For this review, take the finished solid that the model builds, in its own axes (mm). Face numbers are marked on the shaded views. A direction names the side the tool comes from. Round coordinates to 2 decimals unless told otherwise and drop trailing zeros. Order: outer loops, then holes, each group sorted by start corner. A loop starts at its lowest first (then second) coordinate and runs counter-clockwise, first axis right, second up.
from build123d import *

# Parameters (mm, degrees)
BOSS_EXTRUDE1_DEPTH = 13.49375
BOSS_EXTRUDE2_DEPTH = 17.4625


with BuildPart() as part:
    # Sketch1 → Boss-Extrude1 (new body, symmetric)
    with BuildSketch(Plane.XY):
        Polygon((50.8, 0), (-50.8, 0), (-50.8, 34.925), (12.7, 51.939773719), (50.8, 29.942728463), align=None)
    extrude(amount=BOSS_EXTRUDE1_DEPTH, both=True)

    # Sketch2 → Boss-Extrude2 (add)
    with BuildSketch(Plane.XY.offset(13.49375)):
        Polygon((-50.8, 0), (-50.8, 34.925), (0, 21.313181024), (0, 0), align=None)
    extrude(amount=BOSS_EXTRUDE2_DEPTH)


solid = part.part
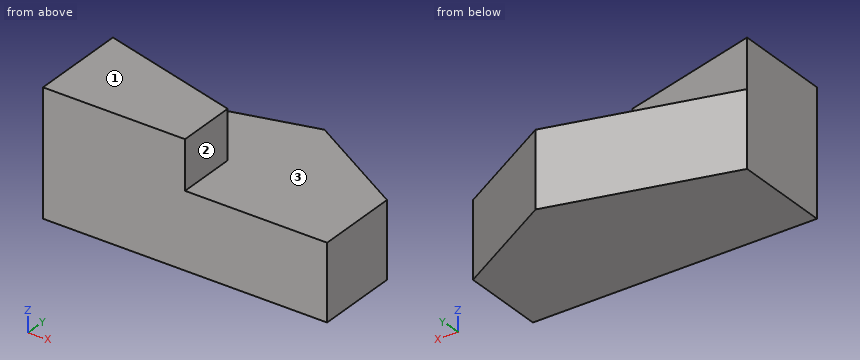
(1) Tool access review of the marked faces 1, 2 and 3: name each direction out of +Z, -Z, +X, -X, +Y, -Y from which nothing blocks a thin tool from reaching the whole face with its end or side.
(2) Add section D-D on x = 15.5. Give the boundary of the cut face in (y, z).
(3) Add section C-C on x = -38. Give the boundary of the cut face in (y, z), plus the area to 3 significant figures.
(4) Clearance check with flat-ended pins moving along their axes: P1, Ø12, axis at y = 39, z = 25.5, coming from the -X side; P2, Ø8.5, axis at y = 7, z = 25, coming from the +X side; P3, Ø10, axis at x = 2.5, y = 30, coming from the +Z side. State where each tip first meets the part, or that it passes through.
(5) Add section B-B on y = 10.5. Give the boundary of the cut face in (x, z), plus the area to 3 significant figures.
(6) Wall thickness on L1, parallel to X at y = 12.5, z = 26.5; L2, parallel to Z at x = 32, y = 11.5; L3, parallel to Y at x = 17.5, z = 13: over which ranges is each line inside the solid? List them lowest first.
(7) Add section A-A on z = -5.5. Give the boundary of the cut face in (x, y) (3 decimals).
Here are the results:
1. face 1: +Z, +X, -X, +Y, -Y
1. face 2: +Z, +X, +Y, -Y
1. face 3: +Z, +X, +Y
2. outline: (0, -13.49) - (50.32, -13.49) - (50.32, 13.49) - (0, 13.49) - close
3. outline: (0, -13.49) - (38.35, -13.49) - (38.35, 13.49) - (31.5, 13.49) - (31.5, 30.96) - (0, 30.96) - close
3. area: 1,590 mm2
4. P1: stops at x = -50.8
4. P2: stops at x = 0
4. P3: stops at z = 13.49
5. outline: (-50.8, -13.49) - (50.8, -13.49) - (50.8, 13.49) - (0, 13.49) - (0, 30.96) - (-50.8, 30.96) - close
5. area: 3,630 mm2
6. L1: x = -50.8 to 0
6. L2: z = -13.49 to 13.49
6. L3: y = 0 to 49.17
7. outline: (-50.8, 0) - (50.8, 0) - (50.8, 29.943) - (12.7, 51.94) - (-50.8, 34.925) - close
